Could you check a few things on this model? Use its own coordinates, in mm. A direction names the side the tool comes from. Round coordinates to 2 decimals unless told otherwise and drop trailing zeros. Write each loop counter-clockwise with the first axis right and the second up, starting at its lowest first coordinate (ties: lowest second). Pieces come first, ordered by that corner, then holes. Notation, with made-up numbers: (74, -36) - (94, -36) arc R17 cw to (94, -30) - close; hole circle Ø7 at (25.25, 82.5). An arc over 180 degrees is marked (long way). Put each result on its own line as item: value.
from build123d import *


with BuildPart() as part:
    # Sketch3 → Revolve1 (revolve)
    with BuildSketch(Plane.XY):
        with BuildLine():
            Line((0, 22.895408163), (0, 0))
            Line((0, 0), (0, -77.104591837))
            Line((0, -77.104591837), (15, -77.104591837))
            Line((15, -77.104591837), (15, -74.104591837))
            ThreePointArc((15, -74.104591837), (6.514718626, -70.589873211), (3, -62.104591837))
            Line((3, -62.104591837), (3, 14.895408163))
            Line((3, 14.895408163), (2, 14.895408163))
            Line((2, 14.895408163), (2, 15.895408163))
            Line((2, 15.895408163), (3, 15.895408163))
            Line((3, 15.895408163), (3, 22.895408163))
            Line((3, 22.895408163), (0, 22.895408163))
        make_face()
    revolve(axis=Axis((0, 103.649150199, 0), (0, -1, 0)))


solid = part.part
(1) For faces 1 (the face through (0, 22.895, 0)), 2 (the face through (-3, 19, 0)), 3 (the face through (-0.434, 15.402, -1.952)), which set-ups out of +Z, -Z, +X, -X, +Y, -Y let a thin tool reach every point of the face, with its end or its side?
Values found:
face 1: +Z, -Z, +X, -X, +Y
face 2: +Y
face 3: none
(2) Please list where these lines run through material, in increasing order: probe 1 along Y at (x, z) = (-10.25, -10.25); probe 2 along Z at (x, y) = (0, -16.5); probe 3 along Z at (x, y) = (3.5, -67). Write a range as from..to.
Values found:
probe 1: y = -77.1..-74.09
probe 2: z = -3..3
probe 3: z = -2.03..2.03
(3) If we mould it in two halves opening along Y, with no side actions, what happens to faces 4 (the face through (0, -77.105, 0)), 5 (the face through (-1, 15.895, -2)), 6 (the face through (-3, -23, 0))? For each: pulls with the +Y half, pulls with the -Y half, needs draft (parallel to the pull), parting line crosses it, or undercut.
Values found:
face 4: pulls with the -Y half
face 5: undercut
face 6: needs draft
(4) Imagine slicing it at B-B, the plane x = 0. List the corners of the cut face in (y, z) for me, then the cut area to 3 significant figures.
Values found:
outline: (-77.1, -15) - (-74.1, -15) arc R12 cw to (-62.1, -3) - (14.9, -3) - (14.9, -2) - (15.9, -2) - (15.9, -3) - (22.9, -3) - (22.9, 3) - (15.9, 3) - (15.9, 2) - (14.9, 2) - (14.9, 3) - (-62.1, 3) arc R12 cw to (-74.1, 15) - (-77.1, 15) - close
area: 732 mm^2
(5) Imagine slicing it at A-A, the plane z = 0. List the corners of the cut face in (x, y) for me.
Values found:
outline: (-15, -77.1) - (15, -77.1) - (15, -74.1) arc R12 cw to (3, -62.1) - (3, 14.9) - (2, 14.9) - (2, 15.9) - (3, 15.9) - (3, 22.9) - (-3, 22.9) - (-3, 15.9) - (-2, 15.9) - (-2, 14.9) - (-3, 14.9) - (-3, -62.1) arc R12 cw to (-15, -74.1) - close
(6) Imagine slicing it at C-C, the plane y = -56.5. List the corners of the cut face in (x, z) for me.
Values found:
outline: circle Ø6 at (0, 0)
(7) I'm going to push flat-ended pins straight in: pin 1 (10 mm diameter, centred on x = -0.5, y = 10, fed in from +Z); pin 2 (1.5 mm diameter, centred on y = 2, z = -3.5, fed in from -X); pin 3 (6 mm diameter, centred on y = -38.5, z = -2.5, fed in from +X). Where does each tip first touch, or does it pass through?
Values found:
pin 1: stops at z = 3
pin 2: stops at x = -1.2
pin 3: stops at x = 3
